Read the model definition and answer for the solid it produces. Units are mm, in the model's axes. Coordinates: 2 decimals unless noted, no trailing zeros. Answer as a JSON object with one key per item and string values. Group by question number.
1) Flat-ended cylindrical pins translate along their axes: P1, Ø1.4, axis at x = 1, z = 262.5, coming from the +Y side; P2, Ø1.4, axis at x = -2, z = 189.5, coming from the -Y side; P3, Ø1.4, axis at y = -1, z = 261, coming from the +X side; P4, Ø2.5, axis at x = 0, y = -20, coming from the +Z side. Find the tip coordinate at first contact, or state that the pin passes through.
2) Section A-A, the plane z = 309 is taken. Count the separate pieces of the cut face and the enclosed holes in it, plus the area to 3 significant figures.
3) Consider probe 1 along Y at (x, z) = (-8.5, 98); probe 2 along Y at (x, z) = (0, 292); probe 3 along X at (y, z) = (-12, 212). Determine where each line is inside the solid, lowest interval first. Write a range as [from, to].
from build123d import *

# Parameters (mm, degrees)
SKETCH1_R           = 2.1
BOSS_EXTRUDE2_DEPTH = 400


with BuildPart() as part:
    # Sketch1 → Boss-Extrude2 (new body)
    with BuildSketch(Plane.XY):
        with BuildLine():
            Line((-8.5, 10), (-4.862792737, 10))
            ThreePointArc((-4.862792737, 10), (-4.598292737, 9.947387679), (-4.374060464, 9.797560464))
            Line((-4.374060464, 9.797560464), (-3.3865, 8.81))
            Line((-3.3865, 8.81), (-3.3865, 8.2))
            Line((-3.3865, 8.2), (-5.5, 8.2))
            Line((-5.5, 8.2), (-5.5, 6.561))
            Line((-5.5, 6.561), (-2.8395, 3.9005))
            Line((-2.8395, 3.9005), (-0.1, 3.9005))
            Line((-0.1, 3.9005), (0, 3.8005))
            Line((0, 3.8005), (0.1, 3.9005))
            Line((0.1, 3.9005), (2.8395, 3.9005))
            Line((2.8395, 3.9005), (5.5, 6.561))
            Line((5.5, 6.561), (5.5, 8.2))
            Line((5.5, 8.2), (3.3865, 8.2))
            Line((3.3865, 8.2), (3.3865, 8.81))
            Line((3.3865, 8.81), (4.374060464, 9.797560464))
            ThreePointArc((4.374060464, 9.797560464), (4.598292737, 9.947387679), (4.862792737, 10))
            Line((4.862792737, 10), (8.5, 10))
            ThreePointArc((8.5, 10), (9.560660172, 9.560660172), (10, 8.5))
            Line((10, 8.5), (10, 4.862792737))
            ThreePointArc((10, 4.862792737), (9.947387679, 4.598292737), (9.797560464, 4.374060464))
            Line((9.797560464, 4.374060464), (8.81, 3.3865))
            Line((8.81, 3.3865), (8.2, 3.3865))
            Line((8.2, 3.3865), (8.2, 5.5))
            Line((8.2, 5.5), (6.561, 5.5))
            Line((6.561, 5.5), (3.9005, 2.8395))
            Line((3.9005, 2.8395), (3.9005, 0.1))
            Line((3.9005, 0.1), (3.8005, 0))
            Line((3.8005, 0), (3.9005, -0.1))
            Line((3.9005, -0.1), (3.9005, -2.8395))
            Line((3.9005, -2.8395), (6.561, -5.5))
            Line((6.561, -5.5), (8.2, -5.5))
            Line((8.2, -5.5), (8.2, -3.3865))
            Line((8.2, -3.3865), (8.81, -3.3865))
            Line((8.81, -3.3865), (9.797560464, -4.374060464))
            ThreePointArc((9.797560464, -4.374060464), (9.947387679, -4.598292737), (10, -4.862792737))
            Line((10, -4.862792737), (10, -15.137207263))
            ThreePointArc((10, -15.137207263), (9.947387679, -15.401707263), (9.797560464, -15.625939536))
            Line((9.797560464, -15.625939536), (8.81, -16.6135))
            Line((8.81, -16.6135), (8.2, -16.6135))
            Line((8.2, -16.6135), (8.2, -14.5))
            Line((8.2, -14.5), (6.561, -14.5))
            Line((6.561, -14.5), (3.9005, -17.1605))
            Line((3.9005, -17.1605), (3.9005, -19.9))
            Line((3.9005, -19.9), (3.8005, -20))
            Line((3.8005, -20), (3.9005, -20.1))
            Line((3.9005, -20.1), (3.9005, -22.8395))
            Line((3.9005, -22.8395), (6.561, -25.5))
            Line((6.561, -25.5), (8.2, -25.5))
            Line((8.2, -25.5), (8.2, -23.3865))
            Line((8.2, -23.3865), (8.81, -23.3865))
            Line((8.81, -23.3865), (9.797560464, -24.374060464))
            ThreePointArc((9.797560464, -24.374060464), (9.947387679, -24.598292737), (10, -24.862792737))
            Line((10, -24.862792737), (10, -28.5))
            ThreePointArc((10, -28.5), (9.560660172, -29.560660172), (8.5, -30))
            Line((8.5, -30), (4.862792737, -30))
            ThreePointArc((4.862792737, -30), (4.598292737, -29.947387679), (4.374060464, -29.797560464))
            Line((4.374060464, -29.797560464), (3.3865, -28.81))
            Line((3.3865, -28.81), (3.3865, -28.2))
            Line((3.3865, -28.2), (5.5, -28.2))
            Line((5.5, -28.2), (5.5, -26.561))
            Line((5.5, -26.561), (2.8395, -23.9005))
            Line((2.8395, -23.9005), (0.1, -23.9005))
            Line((0.1, -23.9005), (0, -23.8005))
            Line((0, -23.8005), (-0.1, -23.9005))
            Line((-0.1, -23.9005), (-2.8395, -23.9005))
            Line((-2.8395, -23.9005), (-5.5, -26.561))
            Line((-5.5, -26.561), (-5.5, -28.2))
            Line((-5.5, -28.2), (-3.3865, -28.2))
            Line((-3.3865, -28.2), (-3.3865, -28.81))
            Line((-3.3865, -28.81), (-4.374060464, -29.797560464))
            ThreePointArc((-4.374060464, -29.797560464), (-4.598292737, -29.947387679), (-4.862792737, -30))
            Line((-4.862792737, -30), (-8.5, -30))
            ThreePointArc((-8.5, -30), (-9.560660172, -29.560660172), (-10, -28.5))
            Line((-10, -28.5), (-10, -24.862792737))
            ThreePointArc((-10, -24.862792737), (-9.947387679, -24.598292737), (-9.797560464, -24.374060464))
            Line((-9.797560464, -24.374060464), (-8.81, -23.3865))
            Line((-8.81, -23.3865), (-8.2, -23.3865))
            Line((-8.2, -23.3865), (-8.2, -25.5))
            Line((-8.2, -25.5), (-6.561, -25.5))
            Line((-6.561, -25.5), (-3.9005, -22.8395))
            Line((-3.9005, -22.8395), (-3.9005, -20.1))
            Line((-3.9005, -20.1), (-3.8005, -20))
            Line((-3.8005, -20), (-3.9005, -19.9))
            Line((-3.9005, -19.9), (-3.9005, -17.1605))
            Line((-3.9005, -17.1605), (-6.561, -14.5))
            Line((-6.561, -14.5), (-8.2, -14.5))
            Line((-8.2, -14.5), (-8.2, -16.6135))
            Line((-8.2, -16.6135), (-8.81, -16.6135))
            Line((-8.81, -16.6135), (-9.797560464, -15.625939536))
            ThreePointArc((-9.797560464, -15.625939536), (-9.947387679, -15.401707263), (-10, -15.137207263))
            Line((-10, -15.137207263), (-10, -4.862792737))
            ThreePointArc((-10, -4.862792737), (-9.947387679, -4.598292737), (-9.797560464, -4.374060464))
            Line((-9.797560464, -4.374060464), (-8.81, -3.3865))
            Line((-8.81, -3.3865), (-8.2, -3.3865))
            Line((-8.2, -3.3865), (-8.2, -5.5))
            Line((-8.2, -5.5), (-6.561, -5.5))
            Line((-6.561, -5.5), (-3.9005, -2.8395))
            Line((-3.9005, -2.8395), (-3.9005, -0.1))
            Line((-3.9005, -0.1), (-3.8005, 0))
            Line((-3.8005, 0), (-3.9005, 0.1))
            Line((-3.9005, 0.1), (-3.9005, 2.8395))
            Line((-3.9005, 2.8395), (-6.561, 5.5))
            Line((-6.561, 5.5), (-8.2, 5.5))
            Line((-8.2, 5.5), (-8.2, 3.3865))
            Line((-8.2, 3.3865), (-8.81, 3.3865))
            Line((-8.81, 3.3865), (-9.797560464, 4.374060464))
            ThreePointArc((-9.797560464, 4.374060464), (-9.947387679, 4.598292737), (-10, 4.862792737))
            Line((-10, 4.862792737), (-10, 8.5))
            ThreePointArc((-10, 8.5), (-9.560660172, 9.560660172), (-8.5, 10))
        make_face()
        Circle(SKETCH1_R, mode=Mode.SUBTRACT)
        with Locations((0, -20)):
            Circle(SKETCH1_R, mode=Mode.SUBTRACT)
        Polygon((-8.2, -12.7), (-8.2, -7.3), (-6.239, -7.3), (-5.5, -6.561), (-2.8395, -3.9005), (-0.1, -3.9005), (0, -3.8005), (0.1, -3.9005), (2.8395, -3.9005), (5.5, -6.561), (6.239, -7.3), (8.2, -7.3), (8.2, -12.7), (6.239, -12.7), (5.5, -13.439), (2.8395, -16.0995), (0.1, -16.0995), (0, -16.1995), (-0.1, -16.0995), (-2.8395, -16.0995), (-5.5, -13.439), (-6.239, -12.7), align=None, mode=Mode.SUBTRACT)
    extrude(amount=BOSS_EXTRUDE2_DEPTH)


solid = part.part
Determined:
{
 "1": {"P1": "y = 3.9", "P2": "y = -23.9", "P3": "x = 3.9", "P4": "through"},
 "2": {"separate pieces": "1", "enclosed holes": "3", "area": "297 mm²"},
 "3": {"probe 1": "[-30, -23.39], [-16.61, -3.39], [3.39, 10]", "probe 2": "[-23.8, -22.1], [-17.9, -16.2], [-3.8, -2.1], [2.1, 3.8]", "probe 3": "[-10, -8.2], [8.2, 10]"}
}
